Can you work these out from the model? Positions are in its coordinate system, mm. A direction names the side the tool comes from. Round coordinates to 2 decimals unless told otherwise and drop trailing zeros. Write each loop counter-clockwise with the first axis right and the second up, starting at its lowest first coordinate (ties: lowest second). Pieces come first, ordered by that corner, then holes. Notation, with made-up numbers: M 30,17 L 37,17 A19 cw 37,24 Z; hole C 50.5,73 d10. An arc over 180 degrees is marked long. Answer as a JSON object with one key per item and string values. Group by question number.
1) Suppose I cut it at B-B, the plane z = 0.8. State how many separate pieces and enclosed holes the cut face has, and give its area (3 significant figures).
2) Suppose I cut it at A-A, the plane x = 0. Write out the boundary of the cut face in (y, z), and give its area (3 significant figures).
3) Please list where these lines run through material, in increasing order: L1, parallel to Y at x = -37, z = 0.9; L2, parallel to Y at x = 105, z = 2.3; L3, parallel to Y at x = 40, z = 0.4. Write a range as [from, to].
4) I'm going to push flat-ended pins straight in: pin 1 Ø1 at (y, z) = (102, 2) entering from -X; pin 2 Ø0.9 at (x, z) = (134, 2) entering from -Y; pin 3 Ø1 at (x, z) = (193, 2) entering from -Y. Where does each tip first touch, or does it pass through?
5) On a 3-axis mill with a long thin cutter (end or side, diameter ignored), from which of +Z, -Z, +X, -X, +Y, -Y can I reach the whole of each face in a straight line? I mean faces 5 (the flat face through (89.2, -204.6, 1.5)), 6 (the flat face through (-3, 133, 3)). Say none if no direction works.
6) If we mould it in two halves opening along X, with no side actions, what happens to faces 1 (the flat face through (-217.964, 38.703, 1.521)), 2 (the flat face through (-176.389, -99.587, 1.479)), 3 (the cylindrical face through (149.154, 199.944, 1.521)), 4 (the flat face through (-221.816, 25.094, 1.521))? For each: +X half, -X half, draft (parallel to the pull), parting line (faces both ways), or undercut.
7) Suppose I cut it at C-C, the plane y = -156. Write out the boundary of the cut face in (x, z).
8) Suppose I cut it at D-D, the plane y = 149.5. Write out the boundary of the cut face in (x, z).
from build123d import *

# Parameters (mm, degrees)
SKETCH_1_R          = 130
SKETCH_1_R_2        = 2
SKETCH_1_R_3        = 2.5
SKETCH_1_R_4        = 1.75
EXTRUDE_1_DEPTH     = 3
SKETCH_8_W          = 20
SKETCH_8_H          = 20
CUT_EXTRUDE_4_DEPTH = 4
FILLET_2_R          = 20


with BuildPart() as part:
    # 草图1 → 凸台-拉伸1 (new body)
    with BuildSketch(Plane.XY):
        Polygon((150.828607906, 202.550991214), (-150.828607906, 202.550991214), (-250.828607906, 29.345910457), (-100, -231.89690167), (100, -231.89690167), (250.828607906, 29.345910457), align=None)
        Circle(SKETCH_1_R, mode=Mode.SUBTRACT)
        with Locations((-199.191349288, 5.907554968)):
            Circle(SKETCH_1_R_2, mode=Mode.SUBTRACT)
        with Locations((-167.168935942, -49.556891928)):
            Circle(SKETCH_1_R_2, mode=Mode.SUBTRACT)
        with Locations((-126.501995314, -119.994099285)):
            Circle(SKETCH_1_R_2, mode=Mode.SUBTRACT)
        with Locations((-94.479581967, -175.458546182)):
            Circle(SKETCH_1_R_2, mode=Mode.SUBTRACT)
        with Locations((199.191349288, 5.907554968)):
            Circle(SKETCH_1_R_2, mode=Mode.SUBTRACT)
        with Locations((167.168935942, -49.556891928)):
            Circle(SKETCH_1_R_2, mode=Mode.SUBTRACT)
        with Locations((126.501995313, -119.994099286)):
            Circle(SKETCH_1_R_2, mode=Mode.SUBTRACT)
        with Locations((94.479581967, -175.458546182)):
            Circle(SKETCH_1_R_2, mode=Mode.SUBTRACT)
        with Locations((104.711767321, 169.550991214)):
            Circle(SKETCH_1_R_2, mode=Mode.SUBTRACT)
        with Locations((40.666940629, 169.550991214)):
            Circle(SKETCH_1_R_2, mode=Mode.SUBTRACT)
        with Locations((-40.666940629, 169.550991214)):
            Circle(SKETCH_1_R_3, mode=Mode.SUBTRACT)
        with Locations((-104.711767321, 169.550991214)):
            Circle(SKETCH_1_R_2, mode=Mode.SUBTRACT)
        with Locations((125, 198.550991214)):
            Circle(SKETCH_1_R_4, mode=Mode.SUBTRACT)
        with Locations((105, 198.550991214)):
            Circle(SKETCH_1_R_4, mode=Mode.SUBTRACT)
        with Locations((-95, 198.550991214)):
            Circle(SKETCH_1_R_4, mode=Mode.SUBTRACT)
        with Locations((-115, 198.550991214)):
            Circle(SKETCH_1_R_4, mode=Mode.SUBTRACT)
    extrude(amount=EXTRUDE_1_DEPTH)

    # 草图8 → 切除-拉伸4 (cut, through all)
    with BuildSketch(Plane.XY.offset(3)):
        with Locations((-132.5, 169.550991214)):
            Rectangle(SKETCH_8_W, SKETCH_8_H)
        Polygon((-209.42521159, 43.633124432), (-226.745719666, 33.633124432), (-216.745719666, 16.312616357), (-199.42521159, 26.312616357), align=None)
        Polygon((-84.245719666, -213.184115646), (-66.92521159, -203.184115646), (-76.92521159, -185.86360757), (-94.245719666, -195.86360757), align=None)
        Polygon((66.92521159, -203.184115646), (84.245719666, -213.184115646), (94.245719666, -195.86360757), (76.92521159, -185.86360757), align=None)
        Polygon((209.42521159, 43.633124432), (199.42521159, 26.312616357), (216.745719666, 16.312616357), (226.745719666, 33.633124432), align=None)
        with Locations((132.5, 169.550991214)):
            Rectangle(SKETCH_8_W, SKETCH_8_H)
    extrude(amount=-CUT_EXTRUDE_4_DEPTH, mode=Mode.SUBTRACT)

    # 圆角2
    fillet_2_edges = [part.edges().sort_by_distance(p)[0] for p in [
        (-150.828607906, 202.550991214, 1.5),
        (150.828607906, 202.550991214, 1.5),
        (250.828607906, 29.345910457, 1.5),
        (100, -231.89690167, 1.5),
        (-100, -231.89690167, 1.5),
        (-250.828607906, 29.345910457, 1.5),
    ]]
    fillet(fillet_2_edges, radius=FILLET_2_R)


solid = part.part
Results:
{
 "1": {"separate pieces": "1", "enclosed holes": "23", "area": "105,000 mm^2"},
 "2": {"outline": "M -231.9,0 L -130,0 L -130,3 L -231.9,3 Z; M 130,0 L 202.55,0 L 202.55,3 L 130,3 Z", "area": "523 mm^2"},
 "3": {"L1": "[-231.9, -124.62], [124.62, 202.55]", "L2": "[-223.13, -76.65], [76.65, 167.57], [171.53, 196.8], [200.3, 202.55]", "L3": "[-231.9, -123.69], [123.69, 167.67], [171.44, 202.55]"},
 "4": {"pin 1": "x = -209.17", "pin 2": "y = -173.79", "pin 3": "y = -71.68"},
 "5": {"face 5": "+Z, -Z", "face 6": "+Z, +X, -X, +Y, -Y"},
 "6": {"face 1": "undercut", "face 2": "-X half", "face 3": "+X half", "face 4": "undercut"},
 "7": {"outline": "M -143.82,0 L 143.82,0 L 143.82,3 L -143.82,3 Z"},
 "8": {"outline": "M -181.46,0 L 181.46,0 L 181.46,3 L -181.46,3 Z"}
}
